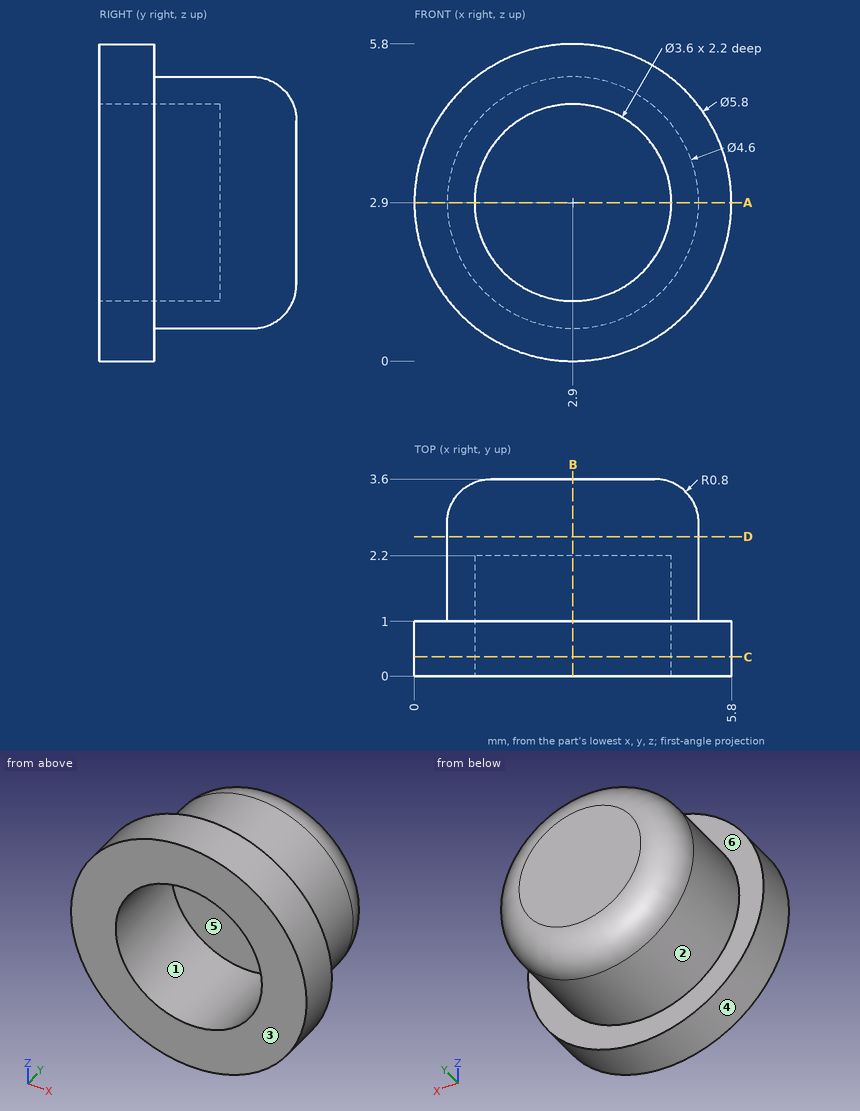
Job drawing, mm, ordinate dimensions from the low corner. One solid piece. A direction names the side the tool comes from. Give positions to 0.01 mm unless a question says otherwise; leave off trailing zeros. Loops run counter-clockwise (first coordinate to the right, second up) from the corner with the lowest first, then second, coordinate; pieces in that order, holes last. Notation, with made-up numbers: M -37,68 L 9,68 A21 ccw 9,96 Z; hole C 1,-13 d10. An arc over 180 degrees is marked long. Answer in a Markdown table with one row per item. Add a question column.
Item 1: Drop a flat-ended pin along its axis: P1, Ø1.1, axis at x = 2, z = 3.5, coming from the -Y side. Give the stop position or say it passes through.
Item 2: Band-saw the part on A-A on z = 2.9. Give the cut face in (x, y).
Item 3: Mould opens along X. For the marked faces 4, 5 and 6 say: +X half, -X half, draft (parallel to the pull), parting line (faces both ways), or undercut.
Item 4: Band-saw the part on B-B on x = 2.9. Give the cut face in (y, z), then the cut area to 3 significant figures.
Item 5: Band-saw the part on C-C on y = 0.35. Give the cut face in (x, z), then the cut area to 3 significant figures.
Item 6: Probe probe 1 along Z at (x, y) = (2.9, 1.7); probe 2 along Z at (x, y) = (2.9, 0.8); probe 3 along Y at (x, z) = (3.4, 1.95). List the from-to ranges inside material, lowest first.
Item 7: Tool access for the marked faces 1, 2 and 3: list every direction of +Z, -Z, +X, -X, +Y, -Y with a clear straight run to the whole face (end or side of a thin tool).
Item 8: Band-saw the part on D-D on y = 2.55. Give the cut face in (x, z).
Reply:
| question | item | result |
|---|---|---|
| 1 | P1 | stops at y = 2.2 |
| 2 | outline | M 0,0 L 1.1,0 L 1.1,2.2 L 4.7,2.2 L 4.7,0 L 5.8,0 L 5.8,1 L 5.2,1 L 5.2,2.8 A0.8 ccw 4.4,3.6 L 1.4,3.6 A0.8 ccw 0.6,2.8 L 0.6,1 L 0,1 Z |
| 3 | face 4 | parting line |
| 3 | face 5 | undercut |
| 3 | face 6 | draft |
| 4 | outline | M 0,0 L 1,0 L 1,0.6 L 2.8,0.6 A0.8 ccw 3.6,1.4 L 3.6,4.4 A0.8 ccw 2.8,5.2 L 1,5.2 L 1,5.8 L 0,5.8 L 0,4.7 L 2.2,4.7 L 2.2,1.1 L 0,1.1 Z |
| 4 | area | 9.57 mm^2 |
| 5 | outline | C 2.9,2.9 d5.8; hole C 2.9,2.9 d3.6 |
| 5 | area | 16.2 mm^2 |
| 6 | probe 1 | z = 0.6 to 1.1, 4.7 to 5.2 |
| 6 | probe 2 | z = 0 to 1.1, 4.7 to 5.8 |
| 6 | probe 3 | y = 2.2 to 3.6 |
| 7 | face 1 | -Y |
| 7 | face 2 | +Y |
| 7 | face 3 | +Z, -Z, +X, -X, -Y |
| 8 | outline | C 2.9,2.9 d4.6 |
